Read the model definition and answer for the solid it produces. Units are mm, in the model's axes. A direction names the side the tool comes from. Give positions to 0.01 mm unless a question says otherwise; leave off trailing zeros. Loops run counter-clockwise (first coordinate to the right, second up) from the corner with the lowest first, then second, coordinate; pieces in that order, holes last. Notation, with made-up numbers: (79, 18) - (118, 18) arc R29 cw to (118, 45) - close; hole circle Ø1 at (-31, 62.5). An arc over 180 degrees is marked (long way). Write item = value, one per line.
```python
from build123d import *

# Parameters (mm, degrees)
F1_W     = 42
F1_H     = 70
F1_R     = 1.6
F1_W_2   = 3
F1_H_2   = 23.75
F2_DEPTH = 2.8
F3_R     = 3
F4_DEPTH = 1.8
F5_R     = 1


with BuildPart() as f2:
    # F1 (on face) → F2 (new body)
    with BuildSketch(Plane.XY):
        Rectangle(F1_W, F1_H)
        with Locations((-16.5, -30.5)):
            Circle(F1_R, mode=Mode.SUBTRACT)
        Polygon((-12, -26), (-1.5, -15.5), (-1.5, -26), align=None, mode=Mode.SUBTRACT)
        with Locations((-16.5, -14.125)):
            Rectangle(F1_W_2, F1_H_2, mode=Mode.SUBTRACT)
        Polygon((-1.5, 0.742641), (-1.5, -11.257359), (-12, -21.757359), (-12, -9.757359), align=None, mode=Mode.SUBTRACT)
        Polygon((1.5, -26), (1.5, -15.5), (12, -26), align=None, mode=Mode.SUBTRACT)
        with Locations((16.5, -30.5)):
            Circle(F1_R, mode=Mode.SUBTRACT)
        Polygon((12, -21.757359), (1.5, -11.257359), (1.5, 0.742641), (12, -9.757359), align=None, mode=Mode.SUBTRACT)
        with Locations((16.5, -14.125)):
            Rectangle(F1_W_2, F1_H_2, mode=Mode.SUBTRACT)
        with Locations((-16.5, 14.125)):
            Rectangle(F1_W_2, F1_H_2, mode=Mode.SUBTRACT)
        Polygon((-1.5, 16.985281), (-1.5, 4.985281), (-12, -5.514719), (-12, 6.485281), align=None, mode=Mode.SUBTRACT)
        with Locations((-16.5, 30.5)):
            Circle(F1_R, mode=Mode.SUBTRACT)
        Polygon((-12, 10.727922), (-12, 26), (-1.5, 26), (-1.5, 21.227922), align=None, mode=Mode.SUBTRACT)
        Polygon((12, -5.514719), (1.5, 4.985281), (1.5, 16.985281), (12, 6.485281), align=None, mode=Mode.SUBTRACT)
        with Locations((16.5, 14.125)):
            Rectangle(F1_W_2, F1_H_2, mode=Mode.SUBTRACT)
        Polygon((1.5, 26), (12, 26), (12, 10.727922), (1.5, 21.227922), align=None, mode=Mode.SUBTRACT)
        with Locations((16.5, 30.5)):
            Circle(F1_R, mode=Mode.SUBTRACT)
    extrude(amount=F2_DEPTH)

    # F3 (on face) → F4 (cut)
    with BuildSketch(Plane.XY.offset(2.8)):
        with Locations((-16.5, -30.5)):
            Circle(F3_R)
        with Locations((16.5, -30.5)):
            Circle(F3_R)
        with Locations((-16.5, 30.5)):
            Circle(F3_R)
        with Locations((16.5, 30.5)):
            Circle(F3_R)
    extrude(amount=-F4_DEPTH, mode=Mode.SUBTRACT)

    # F5
    f5_edges = [f2.edges().sort_by_distance(p)[0] for p in [
        (-15, 14.125, 2.8),
        (15, 14.125, 2.8),
        (-15, -14.125, 2.8),
        (15, -14.125, 2.8),
    ]]
    fillet(f5_edges, radius=F5_R)


solid = f2.part
```
1) A cutting plane is placed at B-B on x = -16.5. Determine the outline of the cut face in (y, z), then the cut area to 3 significant figures.
Output:
outline = (-35, 0) - (-32.1, 0) - (-32.1, 1) - (-33.5, 1) - (-33.5, 2.8) - (-35, 2.8) - close; (-28.9, 0) - (-26, 0) - (-26, 2.8) - (-27.5, 2.8) - (-27.5, 1) - (-28.9, 1) - close; (-2.25, 0) - (2.25, 0) - (2.25, 2.8) - (-2.25, 2.8) - close; (26, 0) - (28.9, 0) - (28.9, 1) - (27.5, 1) - (27.5, 2.8) - (26, 2.8) - close; (32.1, 0) - (35, 0) - (35, 2.8) - (33.5, 2.8) - (33.5, 1) - (32.1, 1) - close
area = 35.0 mm²
2) A cutting plane is placed at D-D on x = -9. Determine the outline of the cut face in (y, z), then the cut area to 3 significant figures.
Output:
outline = (-35, 0) - (-26, 0) - (-26, 2.8) - (-35, 2.8) - close; (-23, 0) - (-18.76, 0) - (-18.76, 2.8) - (-23, 2.8) - close; (-6.76, 0) - (-2.51, 0) - (-2.51, 2.8) - (-6.76, 2.8) - close; (9.49, 0) - (13.73, 0) - (13.73, 2.8) - (9.49, 2.8) - close; (26, 0) - (35, 0) - (35, 2.8) - (26, 2.8) - close
area = 86.0 mm²
3) Each of these flat-tipped pins is pushed along its axis until it touches: P1, Ø3, axis at x = 16.5, y = 30.5, coming from the +Z side; P2, Ø3.5, axis at x = -16.5, y = 30.5, coming from the -Z side. Where does it stop, or does it pass through?
Output:
P1 = through
P2 = 0
4) A cutting plane is placed at C-C on y = -24. Determine the outline of the cut face in (x, z).
Output:
outline = (-21, 0) - (-18, 0) - (-18, 2.8) - (-21, 2.8) - close; (-15, 0) - (-10, 0) - (-10, 2.8) - (-14, 2.8) arc R1 ccw to (-15, 1.8) - close; (-1.5, 0) - (1.5, 0) - (1.5, 2.8) - (-1.5, 2.8) - close; (10, 0) - (15, 0) - (15, 1.8) arc R1 ccw to (14, 2.8) - (10, 2.8) - close; (18, 0) - (21, 0) - (21, 2.8) - (18, 2.8) - close
5) Find the intervals of material crossed by probe 1 along Y at (x, z) = (-16.5, 0.55); probe 2 along Y at (x, z) = (16.5, 1.9); probe 3 along X at (y, z) = (-30.5, 0.4), in increasing order.
Output:
probe_1 = -35 to -32.1, -28.9 to -26, -2.25 to 2.25, 26 to 28.9, 32.1 to 35
probe_2 = -35 to -33.5, -27.5 to -26, -2.25 to 2.25, 26 to 27.5, 33.5 to 35
probe_3 = -21 to -18.1, -14.9 to 14.9, 18.1 to 21
6) The mould has two halves that part along X. Classify faces 4 (the face through (-21, 0, 1)), 5 (the face through (0, 0, 0)), 6 (the face through (-19.5, 30.6, 1.9)): pulls with the +X half, pulls with the -X half, needs draft (parallel to the pull), parting line crosses it, or undercut.
Output:
face_4 = pulls with the -X half
face_5 = needs draft
face_6 = undercut
7) A cutting plane is placed at A-A on y = 30.5. Determine the outline of the cut face in (x, z).
Output:
outline = (-21, 0) - (-18.1, 0) - (-18.1, 1) - (-19.5, 1) - (-19.5, 2.8) - (-21, 2.8) - close; (-14.9, 0) - (14.9, 0) - (14.9, 1) - (13.5, 1) - (13.5, 2.8) - (-13.5, 2.8) - (-13.5, 1) - (-14.9, 1) - close; (18.1, 0) - (21, 0) - (21, 2.8) - (19.5, 2.8) - (19.5, 1) - (18.1, 1) - close
8) A tool of negligible diameter and unlimited length cuts with its end or side. For faces 1 (the face through (12, 1, 1)), 2 (the face through (18, -32, 1)), 3 (the face through (0, 0, 2.8)), from which of +Z, -Z, +X, -X, +Y, -Y can it reach the whole face along a straight path? Write none if from no direction.
Output:
face_1 = +Z, -Z
face_2 = +Z
face_3 = +Z, +X, -X, +Y, -Y
